from build123d import *

# Parameters (mm, degrees)
SHS_RHS50X50X5_1_DEPTH  = 900
CUT_EXTRUDE1_DEPTH      = 452.386752132
CUT_EXTRUDE1_DEPTH_BACK = 452.386752132
SKETCH20_W              = 50
SKETCH20_H              = 40.1
FILLET1_START           = -25
FILLET1_DEPTH           = 5
FILLET1_START_2         = 20
FILLET1_2_DEPTH         = 5
CUT_EXTRUDE2_DEPTH      = 10


with BuildPart() as part:
    # Sketch116 → Shs RHS50X50X5(1) (new body)
    with BuildSketch(Plane.YZ.offset(-450)):
        with BuildLine():
            Line((-15, -25), (15, -25))
            ThreePointArc((15, -25), (22.071067812, -22.071067812), (25, -15))
            Line((25, -15), (25, 15))
            ThreePointArc((25, 15), (22.071067812, 22.071067812), (15, 25))
            Line((15, 25), (-15, 25))
            ThreePointArc((-15, 25), (-22.071067812, 22.071067812), (-25, 15))
            Line((-25, 15), (-25, -15))
            ThreePointArc((-25, -15), (-22.071067812, -22.071067812), (-15, -25))
        make_face()
        with BuildLine():
            Line((-15, -20), (15, -20))
            ThreePointArc((15, -20), (18.535533906, -18.535533906), (20, -15))
            Line((20, -15), (20, 15))
            ThreePointArc((20, 15), (18.535533906, 18.535533906), (15, 20))
            Line((15, 20), (-15, 20))
            ThreePointArc((-15, 20), (-18.535533906, 18.535533906), (-20, 15))
            Line((-20, 15), (-20, -15))
            ThreePointArc((-20, -15), (-18.535533906, -18.535533906), (-15, -20))
        make_face(mode=Mode.SUBTRACT)
    extrude(amount=SHS_RHS50X50X5_1_DEPTH)

    # Sketch20 → Cut-Extrude1 (cut, two sides: drawn at the far end of the back side and taken through both)
    with BuildSketch(Plane(origin=(0, 0, 0), x_dir=(1, 0, 0), z_dir=(0, 1, 0)).offset(-CUT_EXTRUDE1_DEPTH_BACK)):
        with Locations((425, -4.95)):
            Rectangle(SKETCH20_W, SKETCH20_H)
        with Locations((-425, -4.95)):
            Rectangle(SKETCH20_W, SKETCH20_H)
    extrude(amount=CUT_EXTRUDE1_DEPTH + CUT_EXTRUDE1_DEPTH_BACK, mode=Mode.SUBTRACT)

    # Fillet1: read off the stored shape, not the designer's step
    # Fillet1 outline → Fillet1 (add)
    with BuildSketch(Plane(origin=(0, 0, 0), x_dir=(1, 0, 0), z_dir=(0, 1, 0)).offset(FILLET1_START)):
        with BuildLine():
            Line((400, 15.1), (400, 10.1))
            ThreePointArc((400, 10.1), (401.464466094, 13.635533906), (405, 15.1))
            Line((405, 15.1), (400, 15.1))
        make_face()
        with BuildLine():
            Line((-400, 15.1), (-405, 15.1))
            ThreePointArc((-405, 15.1), (-401.464466094, 13.635533906), (-400, 10.1))
            Line((-400, 10.1), (-400, 15.1))
        make_face()
    extrude(amount=FILLET1_DEPTH)

    # Fillet1 2 outline → Fillet1 2 (add)
    with BuildSketch(Plane(origin=(0, 0, 0), x_dir=(1, 0, 0), z_dir=(0, 1, 0)).offset(FILLET1_START_2)):
        with BuildLine():
            Line((400, 15.1), (400, 10.1))
            ThreePointArc((400, 10.1), (401.464466094, 13.635533906), (405, 15.1))
            Line((405, 15.1), (400, 15.1))
        make_face()
        with BuildLine():
            Line((-400, 15.1), (-405, 15.1))
            ThreePointArc((-405, 15.1), (-401.464466094, 13.635533906), (-400, 10.1))
            Line((-400, 10.1), (-400, 15.1))
        make_face()
    extrude(amount=FILLET1_2_DEPTH)

    # Sketch21 → Cut-Extrude2 (cut)
    with BuildSketch(Plane(origin=(0, 0, -25), x_dir=(-1, 0, 0), z_dir=(0, 0, 1))):
        with BuildLine():
            Line((420, 3.25), (430, 3.25))
            ThreePointArc((430, 3.25), (433.25, 0), (430, -3.25))
            Line((430, -3.25), (420, -3.25))
            ThreePointArc((420, -3.25), (416.75, 0), (420, 3.25))
        make_face()
        with BuildLine():
            Line((-430, 3.25), (-420, 3.25))
            ThreePointArc((-420, 3.25), (-416.75, 0), (-420, -3.25))
            Line((-420, -3.25), (-430, -3.25))
            ThreePointArc((-430, -3.25), (-433.25, 0), (-430, 3.25))
        make_face()
    extrude(amount=CUT_EXTRUDE2_DEPTH, mode=Mode.SUBTRACT)


solid = part.part
Can you work these out from the model? Positions are in its coordinate system, mm. A direction names the side the tool comes from. Coordinates: 2 decimals unless noted, no trailing zeros. Write each loop counter-clockwise with the first axis right and the second up, starting at its lowest first coordinate (ties: lowest second). Pieces come first, ordered by that corner, then holes. Notation, with made-up numbers: M 5,72 L 24,72 A30 cw 24,99 Z; hole C -2.75,53 d9. An arc over 180 degrees is marked long. Use one line per item in the form item = value.
Q1. For P1, Ø17.5, axis at y = -5.5, z = 13, coming from the +X side; P2, Ø2.5, axis at x = 413, y = -22.5, coming from the +Z side; P3, Ø10, axis at x = 175.5, z = -20, coming from the +Y side; P4, Ø1.5, axis at x = 426, z = -23.5, coming from the +Y side, each with a flat end and sliding along its axis, tell me the tip position at first contact or that it passes through.
Model answer:
P1 = 400
P2 = -15.1
P3 = 25
P4 = 21.32
Q2. I need wall thicknesses on line 1 along Z through (x, y) = (113, 11); line 2 along Z through (x, y) = (-99, -16.5). Which ranges of each line are inside material? Lowest first, please. Write a range as from..to.
Model answer:
line_1 = -25..-20, 20..25
line_2 = -24.89..-19.77, 19.77..24.89
Q3. If we section it at A-A (x = -5.5): Write out the boundary of the cut face in (y, z), then the cut area to 3 significant figures.
Model answer:
outline = M -25,-15 A10 ccw -15,-25 L 15,-25 A10 ccw 25,-15 L 25,15 A10 ccw 15,25 L -15,25 A10 ccw -25,15 Z; hole M -20,-15 A5 ccw -15,-20 L 15,-20 A5 ccw 20,-15 L 20,15 A5 ccw 15,20 L -15,20 A5 ccw -20,15 Z
area = 836 mm^2
Q4. We'd pull the mould along Z, two halves only. Please class faces 1 (the flat face through (-6, -20, 0)), 2 (the flat face through (400, -2, 21)), 3 (the flat face through (-6, 0, -25)), 4 (the flat face through (-6, 0, -20)): +Z half, -Z half, draft (parallel to the pull), parting line (faces both ways), or undercut.
Model answer:
face_1 = undercut
face_2 = draft
face_3 = -Z half
face_4 = undercut
Q5. For faces 5 (the flat face through (-400, -2, 21)), 6 (the flat face through (-6, 0, 20)), 7 (the flat face through (-6, 25, 0)), which set-ups out of +Z, -Z, +X, -X, +Y, -Y let a thin tool reach every point of the face, with its end or its side?
Model answer:
face_5 = +Z, -X, +Y, -Y
face_6 = +X, -X
face_7 = +Z, -Z, +X, -X, +Y
